```python
from build123d import *

# Parameters (mm, degrees)
PLATE_DEPTH                          = 6.35
FILLET1_R                            = 10
TRIPOD_SOCKET_TAP_DRILL_FOR_1_4_20_D = 5.1054
CAMERA_MOUNT_SCREW_CLEARANCE_DEPTH   = 352.602633461
ALIGNMENT_TAP_DRILL_FOR_M2_5_D       = 2.05
CLAMP_TAP_DRILL_FOR_M2_5_D           = 2.05
SKETCH11_R                           = 2.38125
CABLE_TIES_HOLES_DEPTH               = 352.602633461


with BuildPart() as part:
    # Sketch1 → plate (new body)
    with BuildSketch(Plane(origin=(0, 0, 0), x_dir=(1, 0, 0), z_dir=(0, 1, 0))):
        Polygon((13.637433785, 0), (183.637433785, 0), (183.637433785, -300), (13.637433785, -296.115361978), align=None)
    extrude(amount=PLATE_DEPTH)

    # Fillet1
    fillet1_edges = [part.edges().sort_by_distance(p)[0] for p in [
        (13.637433785, 3.175, 0),
        (183.637433785, 3.175, 0),
        (183.637433785, 3.175, 300),
        (13.637433785, 3.175, 296.115361978),
    ]]
    fillet(fillet1_edges, radius=FILLET1_R)

    # tripod socket Tap Drill for 1/4-20 (through all)
    with Locations(Plane(origin=(0, 0, 0), x_dir=(-1, 0, 0), z_dir=(0, -1, 0))):
        with Locations((-98.637433785, -50), (-98.637433785, -125), (-98.637433785, -200)):
            Hole(TRIPOD_SOCKET_TAP_DRILL_FOR_1_4_20_D / 2)

    # Sketch6 → camera mount screw clearance (cut, through all)
    with BuildSketch(Plane(origin=(0, 6.35, 0), x_dir=(1, 0, 0), z_dir=(0, 1, 0))):
        with BuildLine():
            Line((130.137433785, -26.845059814), (130.137433785, -11.845059814))
            ThreePointArc((130.137433785, -11.845059814), (134.637433785, -7.345059814), (139.137433785, -11.845059814))
            Line((139.137433785, -11.845059814), (139.137433785, -26.845059814))
            ThreePointArc((139.137433785, -26.845059814), (134.637433785, -31.345059814), (130.137433785, -26.845059814))
        make_face()
        with BuildLine():
            Line((58.137433785, -26.845059814), (58.137433785, -11.845059814))
            ThreePointArc((58.137433785, -11.845059814), (62.637433785, -7.345059814), (67.137433785, -11.845059814))
            Line((67.137433785, -11.845059814), (67.137433785, -26.845059814))
            ThreePointArc((67.137433785, -26.845059814), (62.637433785, -31.345059814), (58.137433785, -26.845059814))
        make_face()
    extrude(amount=-CAMERA_MOUNT_SCREW_CLEARANCE_DEPTH, mode=Mode.SUBTRACT)

    # alignment Tap Drill for M2.5 (through all)
    with Locations(Plane(origin=(0, 6.35, 0), x_dir=(1, 0, 0), z_dir=(0, 1, 0))):
        with Locations((60.027433785, -82.595059814), (137.247433785, -82.595059814), (137.247433785, -130.855059814), (60.027433785, -130.855059814)):
            Hole(ALIGNMENT_TAP_DRILL_FOR_M2_5_D / 2)

    # clamp Tap Drill for M2.5 (through all)
    with Locations(Plane(origin=(0, 6.35, 0), x_dir=(1, 0, 0), z_dir=(0, 1, 0))):
        with Locations((31.137433785, -70.35), (166.029512109, -70.453390828)):
            Hole(CLAMP_TAP_DRILL_FOR_M2_5_D / 2)

    # Sketch11 → cable ties holes (cut, through all)
    with BuildSketch(Plane(origin=(0, 6.35, 0), x_dir=(1, 0, 0), z_dir=(0, 1, 0))):
        with Locations(Location((33.408985301, -286.564547525, 0), (0, 0, 270))):
            Circle(SKETCH11_R)
        with Locations(Location((43.408985301, -286.564547525, 0), (0, 0, 270))):
            Circle(SKETCH11_R)
        with Locations(Location((153.426530966, -286.648872752, 0), (0, 0, 270))):
            Circle(SKETCH11_R)
        with Locations(Location((163.426519217, -286.664202157, 0), (0, 0, 270))):
            Circle(SKETCH11_R)
    extrude(amount=-CABLE_TIES_HOLES_DEPTH, mode=Mode.SUBTRACT)


solid = part.part
```
Build history of the part. All positions in model axes, mm. A direction names the side the tool comes from. Round coordinates to 2 decimals unless told otherwise and drop trailing zeros. Order: outer loops, then holes, each group sorted by start corner. A loop starts at its lowest first (then second) coordinate and runs counter-clockwise, first axis right, second up. Notation, with made-up numbers: (-18.75, 72) -> (32.25, 72) arc R20 ccw to (32.25, 109) -> close; hole circle Ø4 at (67, 77.5). An arc over 180 degrees is marked (long way). Answer in a Markdown table with one row per item.
1) Wall check: L1, parallel to X at y = 5, z = 21; L2, parallel to X at y = 2.25, z = 70.35; L3, parallel to X at y = 3.5, z = 125. Give the ranges that are in metal, low to high.
Values:
| item | result |
|---|---|
| L1 | 13.64 to 58.14, 67.14 to 130.14, 139.14 to 183.64 |
| L2 | 13.64 to 30.11, 32.16 to 165.01, 167.05 to 183.64 |
| L3 | 13.64 to 96.08, 101.19 to 183.64 |
2) Mould opens along X. For faces 3 (the flat face through (98, 3, 0)), 4 (the flat face through (67.137, 3, 19)), 5 (the flat face through (13.637, 3, 150)) say: released by +X, released by -X, zero draft, split by the parting line, or undercut.
Values:
| item | result |
|---|---|
| face 3 | zero draft |
| face 4 | undercut |
| face 5 | released by -X |
3) Pin check, flat tip, straight feed: P1, Ø4.5, axis at x = 153.43, z = 286.65, coming from the +Y side. Stop position of the tip, or through.
Values:
| item | result |
|---|---|
| P1 | through |
4) Band-saw the part on B-B on y = 2.5. Give the number of separate pieces and of enclosed holes in the cut face, and give its area (3 significant figures).
Values:
| item | result |
|---|---|
| separate pieces | 1 |
| enclosed holes | 15 |
| area | 50,000 mm2 |
5) Which spindle directions (+Z, -Z, +X, -X, +Y, -Y) get a long thin tool onto all of the face, cutting with end or side? Do faces 1 (the cylindrical face through (16.562, 3.219, 293.408)), 2 (the cylindrical face through (62.736, 3.219, 31.344)). Say none if no direction does.
Values:
| item | result |
|---|---|
| face 1 | +Z, -X, +Y, -Y |
| face 2 | +Y, -Y |
6) Band-saw the part on A-A on z = 19. Give the cut face in (x, y).
Values:
| item | result |
|---|---|
| outline | (13.64, 0) -> (58.14, 0) -> (58.14, 6.35) -> (13.64, 6.35) -> close; (67.14, 0) -> (130.14, 0) -> (130.14, 6.35) -> (67.14, 6.35) -> close; (139.14, 0) -> (183.64, 0) -> (183.64, 6.35) -> (139.14, 6.35) -> close |
